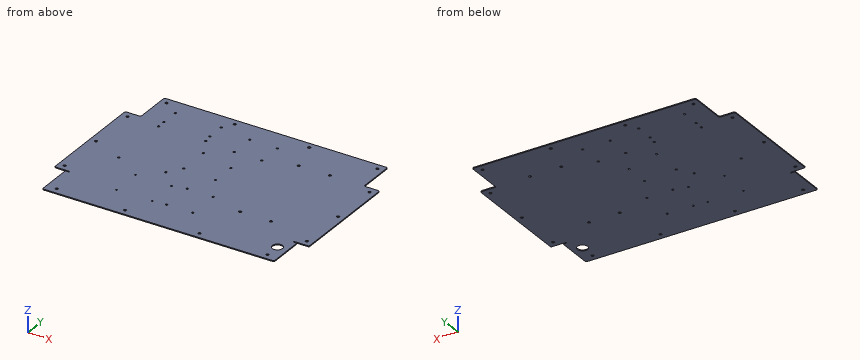
Autodesk Inventor part; units mm, degrees
ref_plane "YZ Plane" through (0, 0, 0) normal (1, 0, 0) x (0, 1, 0)
ref_plane "XZ Plane" through (0, 0, 0) normal (0, 1, 0) x (-1, 0, 0)
ref_plane "XY Plane" through (0, 0, 0) normal (0, 0, 1) x (1, 0, 0)
sketch "スケッチ1" plane through (0, 0, 0) normal (0, 0, 1) x (1, 0, 0)
  circle A0 centre (380.0191, 230.2191) radius 2.25
  circle A1 centre (380.0191, 70.2191) radius 2.25
  circle A2 centre (380.0191, 150.2191) radius 2.25
  circle A3 centre (124.8, 290.4382) radius 2.25
  circle A4 centre (14.8, 290.4382) radius 2.25
  circle A5 centre (354.8, 290.4382) radius 2.25
  circle A6 centre (244.8, 290.4382) radius 2.25
  circle A7 centre (259.8, 240.2191) radius 2.25
  circle A8 centre (259.8, 90.2191) radius 2.25
  circle A9 centre (309.8, 90.2191) radius 2.25
  circle A10 centre (309.8, 240.2191) radius 2.25
  circle A11 centre (116.1, 128.3691) radius 1.75
  circle A12 centre (39.8, 230.2191) radius 1.75
  circle A13 centre (116.1, 230.2191) radius 1.75
  circle A14 centre (39.8, 128.3691) radius 1.75
  circle A15 centre (131.1, 150.2191) radius 1.75
  circle A16 centre (131.1, 200.2191) radius 1.75
  circle A17 centre (164.8, 105.2191) radius 1.75
  circle A18 centre (206.8, 53.2191) radius 1.75
  circle A19 centre (206.8, 105.2191) radius 1.75
  circle A20 centre (164.8, 53.2191) radius 1.75
  circle A21 centre (209.4, 265.2191) radius 1.75
  circle A22 centre (164.8, 225.4191) radius 1.75
  circle A23 centre (164.8, 265.2191) radius 1.75
  circle A24 centre (209.4, 225.4191) radius 1.75
  circle A25 centre (84.8, 51.2191) radius 1.4
  circle A26 centre (142.8, 51.2191) radius 1.4
  circle A27 centre (142.8, 100.2191) radius 1.4
  circle A28 centre (84.8, 100.2191) radius 1.4
  circle A29 centre (39.8, 273.2191) radius 1.75
  circle A30 centre (114, 244.0191) radius 1.75
  circle A31 centre (114, 273.2191) radius 1.75
  circle A32 centre (39.8, 244.0191) radius 1.75
  circle A33 centre (184.8, 146.1191) radius 1.75
  circle A34 centre (184.8, 185.2191) radius 1.75
  circle A35 centre (354.8, 35.2191) radius 8.25
  circle A36 centre (-10.4191, 150.2191) radius 2.25
  circle A37 centre (-10.4191, 70.2191) radius 2.25
  circle A38 centre (-10.4191, 230.2191) radius 2.25
  circle A39 centre (244.8, 10) radius 2.25
  circle A40 centre (354.8, 10) radius 2.25
  circle A41 centre (14.8, 10) radius 2.25
  circle A42 centre (124.8, 10) radius 2.25
  arc A43 (-2, 2) -> (0, 0) centre (0, 2) ccw
  line L0 (369.6, 0) -> (0, 0)
  arc A44 (369.6, 0) -> (371.6, 2) centre (369.6, 2) ccw
  line L1 (371.6, 2) -> (371.6, 56.2191)
  arc A45 (371.6, 56.2191) -> (369.6, 58.2191) centre (369.6, 56.2191) ccw
  line L2 (369.6, 58.2191) -> (365.6, 58.2191)
  line L3 (365.6, 58.2191) -> (365.6, 60.2191)
  line L4 (365.6, 60.2191) -> (388.0191, 60.2191)
  arc A46 (388.0191, 60.2191) -> (390.0191, 62.2191) centre (388.0191, 62.2191) ccw
  line L5 (390.0191, 238.2191) -> (390.0191, 62.2191)
  arc A47 (390.0191, 238.2191) -> (388.0191, 240.2191) centre (388.0191, 238.2191) ccw
  line L6 (388.0191, 240.2191) -> (366.8, 240.2191)
  arc A48 (364.8, 242.2191) -> (366.8, 240.2191) centre (366.8, 242.2191) ccw
  line L7 (364.8, 242.2191) -> (364.8, 298.4382)
  arc A49 (364.8, 298.4382) -> (362.8, 300.4382) centre (362.8, 298.4382) ccw
  line L8 (6.8, 300.4382) -> (362.8, 300.4382)
  arc A50 (6.8, 300.4382) -> (4.8, 298.4382) centre (6.8, 298.4382) ccw
  line L9 (4.8, 298.4382) -> (4.8, 242.2191)
  arc A51 (2.8, 240.2191) -> (4.8, 242.2191) centre (2.8, 242.2191) ccw
  line L10 (2.8, 240.2191) -> (-18.4191, 240.2191)
  arc A52 (-18.4191, 240.2191) -> (-20.4191, 238.2191) centre (-18.4191, 238.2191) ccw
  line L11 (-20.4191, 62.2191) -> (-20.4191, 238.2191)
  arc A53 (-20.4191, 62.2191) -> (-18.4191, 60.2191) centre (-18.4191, 62.2191) ccw
  line L12 (-18.4191, 60.2191) -> (4, 60.2191)
  line L13 (4, 60.2191) -> (4, 58.2191)
  line L14 (4, 58.2191) -> (0, 58.2191)
  arc A54 (0, 58.2191) -> (-2, 56.2191) centre (0, 56.2191) ccw
  line L15 (-2, 56.2191) -> (-2, 2)
extrude "押し出し1" add sketch "スケッチ1" along normal blind 1.6
properties part number "Board_Mount_Flat"
Source: CAD feature listing. Evaluate the final solid. Frame: model axes, mm. Round coordinates to 2 decimals unless told otherwise and drop trailing zeros. Answer as a JSON object with one key per item and string values. Group by question number.
(1) Ray query, line 1 (Y direction, x = 309.8, z = 1.1); line 2 (Y direction, x = 244.8, z = 0.8); line 3 (X direction, y = 230.5, z = 1.4). Return the intervals inside material, ascending. Write a range as [from, to].
(2) First-contact query: pin 1 (0.8 mm diameter, centred on x = -4, z = 1, fed in from -Y). Flat tip, straight axial feed; report the tip coordinate or a pass-through.
(3) Section query A-A on z = 0.85. State how many separate pieces and enclosed holes the cut face has, then the cut area to 3 significant figures.
Computed values:
{
 "1": {"line 1": "[0, 87.97], [92.47, 237.97], [242.47, 300.44]", "line 2": "[0, 7.75], [12.25, 288.19], [292.69, 300.44]", "line 3": "[-20.42, -12.65], [-8.19, 38.07], [41.53, 114.37], [117.83, 377.79], [382.25, 390.02]"},
 "2": {"pin 1": "y = 60.22"},
 "3": {"separate pieces": "1", "enclosed holes": "43", "area": "117,000 mm^2"}
}
